Autodesk Inventor part; units mm, degrees
ref_plane "YZ Plane" through (0, 0, 0) normal (1, 0, 0) x (0, 1, 0)
ref_plane "XZ Plane" through (0, 0, 0) normal (0, 1, 0) x (-1, 0, 0)
ref_plane "XY Plane" through (0, 0, 0) normal (0, 0, 1) x (1, 0, 0)
sketch "Sketch1" plane through (0, 0, 0) normal (0, 1, 0) x (-1, 0, 0)
  line L0 (30, 30) -> (-30, 30)
  line L1 (-30, 30) -> (-30, -30)
  line L2 (-30, -30) -> (30, -30)
  line L3 (30, -30) -> (30, 30)
  point P0 (0, 0)
  point P1 (30, 0)
  point P2 (0, 30)
  dimension "d0" = 60
  dimension "d1" = 60
extrude "Extrusion1" add sketch "Sketch1" along normal blind 0.96
sketch "Sketch2" plane through (0, 0.96, 0) normal (0, 1, 0) x (1, 0, 0)
  line L0 (30, -30) -> (30, 30)
  line L1 (30, 30) -> (-30, 30)
  line L2 (-30, 30) -> (-30, -30)
  line L3 (-30, -30) -> (30, -30)
  line L4 (-30, 0) -> (30, 0)
  line L5 (0, -30) -> (0, 30)
  circle A0 centre (-10.5, -10.5) radius 4.25
  circle A1 centre (-10.5, 10.5) radius 4.25
  circle A2 centre (10.5, 10.5) radius 4.25
  circle A3 centre (10.5, -10.5) radius 4.25
  point P0 (0, 0)
  dimension "d13" = 8.5
  dimension "d14" = 21
  dimension "d15" = 21
extrude "Extrusion2" add sketch "Sketch2" along normal blind 1.92
sketch "Sketch3" plane through (0, 2.88, 0) normal (0, 1, 0) x (1, 0, 0)
  line L0 (-30, 30) -> (-30, -30)
  line L1 (-30, -30) -> (30, -30)
  line L2 (30, -30) -> (30, 30)
  line L3 (30, 30) -> (-30, 30)
  point P0 (0, 0)
extrude "Extrusion3" add sketch "Sketch3" along normal blind 0.64
fillet "Fillet1" radius 8 4 edges at (30, 1.76, 30) (-30, 1.76, 30) (-30, 1.76, -30) (30, 1.76, -30)
ref_plane "Arbeitsebene2" through (27.6569, 3.52, -27.6569) normal (-0.7071, 0, -0.7071) x (0, -1, 0)
sketch "Skizze7" plane through (0, 3.52, 0) normal (0, 1, 0) x (1, 0, 0)
  line L0 (-22, -30) -> (22, -30)
  arc A0 (22, -30) -> (30, -22) centre (22, -22) ccw
  line L1 (30, -22) -> (30, 22)
  arc A1 (30, 22) -> (22, 30) centre (22, 22) ccw
  line L2 (22, 30) -> (-22, 30)
  arc A2 (-22, 30) -> (-30, 22) centre (-22, 22) ccw
  line L3 (-30, 22) -> (-30, -22)
  arc A3 (-30, -22) -> (-22, -30) centre (-22, -22) ccw
  line L4 (22, -30) -> (-22, -30)
  line L5 (-30, -22) -> (-30, 22)
  line L6 (-22, 30) -> (22, 30)
  line L7 (30, 22) -> (30, -22)
  arc A4 (22, -30) -> (30, -22) centre (22, -22) ccw
  arc A5 (-30, -22) -> (-22, -30) centre (-22, -22) ccw
  arc A6 (-22, 30) -> (-30, 22) centre (-22, 22) ccw
  arc A7 (30, 22) -> (22, 30) centre (22, 22) ccw
  point P0 (0, 0)
extrude "Extrusion4" add sketch "Skizze7" along normal blind 3.2
sketch "Skizze8" plane through (0, 6.72, 0) normal (0, 1, 0) x (1, 0, 0)
  line L0 (23.5, 23.5) -> (-23.5, 23.5)
  line L1 (-23.5, 23.5) -> (-23.5, -23.5)
  line L2 (-23.5, -23.5) -> (23.5, -23.5)
  line L3 (23.5, -23.5) -> (23.5, 23.5)
  line L4 (23.5, 23.5) -> (-23.5, -23.5) construction
  line L5 (-23.5, 23.5) -> (23.5, -23.5) construction
  point P0 (0, 0)
  dimension "d25" = 47
  dimension "d26" = 47
extrude "Extrusion5" cut sketch "Skizze8" against normal blind 3.2
chamfer "Fasen2" distance 5 distance2 5.76 8 edges at (0, 6.72, -30) (-27.6569, 6.72, -27.6569) (-30, 6.72, 0) (-27.6569, 6.72, 27.6569) (0, 6.72, 30) (27.6569, 6.72, 27.6569) (30, 6.72, 0) (27.6569, 6.72, -27.6569) measured on face at (7.3333, 6.72, -25.6667)
properties part number "IMU_Base_T-Shirt"
Source: CAD feature listing. Evaluate the final solid. Frame: model axes, mm. A direction names the side the tool comes from. Give positions to 0.01 mm unless a question says otherwise; leave off trailing zeros. Order: outer loops, then holes, each group sorted by start corner. A loop starts at its lowest first (then second) coordinate and runs counter-clockwise, first axis right, second up.
(1) Material intervals for line 1 along Z through (x, y) = (10.5, 1.8); line 2 along Y through (x, z) = (8.5, 8); line 3 along X through (y, z) = (2, 10.5), sorted ascending.
(2) Section query B-B (x = -4.5). Return the cut outline in (y, z), plus the area to 3 significant figures.
(3) Section query A-A (x = 10.5). Return the cut outline in (y, z), plus the area to 3 significant figures.
(4) Contact query for flat-ended pins moving along their axis: P1, Ø4, axis at x = 12, z = 9, coming from the +Y side; P2, Ø3.5, axis at y = 4.5, z = -11, coming from the +X side; P3, Ø2.5, axis at x = -10.5, y = 4.5, coming from the -Z side. Output: stop coordinate, or through.
(5) Access query for faces 1 (the face through (-27.594, 0.473, 27.719)), 2 (the face through (11, 0.96, -10)), 3 (the face through (0, 3.52, 0)). Directions: +Z, -Z, +X, -X, +Y, -Y. A direction counts if a zero-diameter tool reaches every point of the face in a straight line with its end or side. Return the directions, or none.
(6) Section query D-D (z = -18). Return the cut outline in (x, y).
(7) Section query C-C (z = 10.5). Return the cut outline in (x, y), plus the area to 3 significant figures.
(8) Pull-direction query (Z, two-part tool) for faces 4 (the face through (-25.96, 3.8, -25.87)), 5 (the face through (25.96, 3.8, 25.87)), 6 (the face through (-10, 0.96, -10)); classes: +Z half, -Z half, draft (parallel to the pull), parting line (faces both ways), or undercut.
Outcome:
1. line 1: z = -29.27 to -14.75, -6.25 to 6.25, 14.75 to 29.27
1. line 2: y = 0 to 0.96, 2.88 to 3.52
1. line 3: x = -29.1 to -14.75, -6.25 to 6.25, 14.75 to 29.1
2. outline: (0, -30) - (0.96, -30) - (6.72, -25) - (6.72, -23.5) - (3.52, -23.5) - (3.52, 23.5) - (6.72, 23.5) - (6.72, 25) - (0.96, 30) - (0, 30) - close
2. area: 224 mm2
3. outline: (0, -30) - (0.96, -30) - (6.72, -25) - (6.72, -23.5) - (3.52, -23.5) - (3.52, 23.5) - (6.72, 23.5) - (6.72, 25) - (0.96, 30) - (0, 30) - close; hole (0.96, -14.75) - (2.88, -14.75) - (2.88, -6.25) - (0.96, -6.25) - close; hole (0.96, 6.25) - (2.88, 6.25) - (2.88, 14.75) - (0.96, 14.75) - close
3. area: 191 mm2
4. P1: stops at y = 3.52
4. P2: stops at x = 28.45
4. P3: stops at z = -28.01
5. face 1: +Z, -X, +Y, -Y
5. face 2: none
5. face 3: +Y
6. outline: (-30, 0) - (30, 0) - (30, 0.96) - (25, 6.72) - (23.5, 6.72) - (23.5, 3.52) - (-23.5, 3.52) - (-23.5, 6.72) - (-25, 6.72) - (-30, 0.96) - close
7. outline: (-30, 0) - (30, 0) - (30, 0.96) - (25, 6.72) - (23.5, 6.72) - (23.5, 3.52) - (-23.5, 3.52) - (-23.5, 6.72) - (-25, 6.72) - (-30, 0.96) - close; hole (-14.75, 0.96) - (-6.25, 0.96) - (-6.25, 2.88) - (-14.75, 2.88) - close; hole (6.25, 0.96) - (14.75, 0.96) - (14.75, 2.88) - (6.25, 2.88) - close
7. area: 191 mm2
8. face 4: -Z half
8. face 5: +Z half
8. face 6: undercut
